from build123d import *

# Parameters (mm, degrees)
F0_W     = 83.383921
F0_H     = 73.864564
F1_DEPTH = 25.4
F2_R     = 7.62
F3_R     = 12.7
F4_DEPTH = 25.4
F5_R     = 5.08


with BuildPart() as f1:
    # F0 (on Front) → F1 (new body, symmetric)
    with BuildSketch(Plane.XZ):
        with Locations((-8.381387, 24.481572)):
            Rectangle(F0_W, F0_H)
    extrude(amount=F1_DEPTH, both=True)

    # F2
    f2_edges = [f1.edges().sort_by_distance(p)[0] for p in [
        (-50.073348, 0, -12.45071),
        (33.310573, 0, -12.45071),
        (33.310573, 0, 61.413854),
        (-50.073348, 0, 61.413854),
        (-50.073348, 25.4, 24.481572),
        (-50.073348, -25.4, 24.481572),
        (-8.381388, 25.4, 61.413854),
        (-8.381388, 25.4, -12.45071),
        (33.310573, 25.4, 24.481572),
        (-8.381388, -25.4, 61.413854),
        (-8.381388, -25.4, -12.45071),
        (33.310573, -25.4, 24.481572),
    ]]
    fillet(f2_edges, radius=F2_R)

    # F3 (on face) → F4 (join)
    with BuildSketch(Plane(origin=(0, 25.4, 0), x_dir=(-1, 0, 0), z_dir=(0, 1, 0))):
        with Locations((-8.346652, 31.472079)):
            Circle(F3_R)
    extrude(amount=F4_DEPTH)

    # F5
    f5_edges = [f1.edges().sort_by_distance(p)[0] for p in [
        (21.046652, 50.8, 31.472079),
    ]]
    fillet(f5_edges, radius=F5_R)


solid = f1.part
Model file for the job. Use its own axes, mm. A direction names the side the tool comes from. Round coordinates to 2 decimals unless told otherwise and drop trailing zeros. Loops run counter-clockwise (first coordinate to the right, second up) from the corner with the lowest first, then second, coordinate; pieces in that order, holes last.
1. Band-saw the part on C-C, the plane y = 39. List the corners of the cut face in (x, z).
Check values:
outline: circle Ø25.4 at (8.35, 31.47)
2. Tool access for faces 1 (the cylindrical face through (2.5, 35.4, 20.2)), 2 (the flat face through (-50.073, 0, 24)): list every direction of +Z, -Z, +X, -X, +Y, -Y with a clear straight run to the whole face (end or side of a thin tool).
Check values:
face 1: +Y
face 2: +Z, -Z, -X, +Y, -Y
3. Drop flat-ended pins along their axis: P1, Ø8, axis at x = -13.5, y = 22, coming from the +Z side; P2, Ø3, axis at x = -23, z = 35, coming from the +Y side; P3, Ø12, axis at x = 7.5, z = 20, coming from the +Y side; P4, Ø2, axis at x = -4, y = 39.5, coming from the -Z side. Give the stop position or say it passes through.
Check values:
P1: stops at z = 61.41
P2: stops at y = 25.4
P3: stops at y = 50.8
P4: stops at z = 25.77
4. Band-saw the part on B-B, the plane z = 16.5. List the corners of the cut face in (x, y), and give its area (3 significant figures).
Check values:
outline: (-50.07, -17.78) arc R7.62 ccw to (-42.45, -25.4) - (25.69, -25.4) arc R7.62 ccw to (33.31, -17.78) - (33.31, 17.78) arc R7.62 ccw to (25.69, 25.4) - (-42.45, 25.4) arc R7.62 ccw to (-50.07, 17.78) - close
area: 4,190 mm2
5. Band-saw the part on A-A, the plane x = -37.5. List the corners of the cut face in (y, z), and give its area (3 significant figures).
Check values:
outline: (-25.4, -4.83) arc R7.62 ccw to (-17.78, -12.45) - (17.78, -12.45) arc R7.62 ccw to (25.4, -4.83) - (25.4, 53.79) arc R7.62 ccw to (17.78, 61.41) - (-17.78, 61.41) arc R7.62 ccw to (-25.4, 53.79) - close
area: 3,700 mm2
6. Wall check: probe 1 along Y at (x, z) = (-6.5, 38); probe 2 along X at (y, z) = (30, 39); probe 3 along Z at (x, y) = (3.5, -21). Give the ranges that are in metal, low to high.
Check values:
probe 1: y = -25.4 to 25.4
probe 2: x = -1.88 to 18.58
probe 3: z = -11.74 to 60.7
